Can you work these out from the model? Positions are in its coordinate system, mm. A direction names the side the tool comes from. Coordinates: 2 decimals unless noted, no trailing zeros. Write each loop counter-clockwise with the first axis right and the second up, starting at its lowest first coordinate (ties: lowest second). Pieces come first, ordered by that corner, then holes.
```python
from build123d import *

# Parameters (mm, degrees)
SKETCH1_W                      = 69.85
SKETCH1_H                      = 44.45
BOSS_EXTRUDE1_DEPTH            = 3.175
BOSS_EXTRUDE2_DEPTH            = 5.08
FILLET1_R                      = 6.35
F_6_0_204_DIAMETER_HOLE1_D     = 3.6576
F_6_0_204_DIAMETER_HOLE1_DEPTH = 38.1
F_6_0_204_DIAMETER_HOLE1_TIP   = 1.0988539


with BuildPart() as part:
    # Sketch1 → Boss-Extrude1 (new body)
    with BuildSketch(Plane(origin=(0, 0, 0), x_dir=(1, 0, 0), z_dir=(0, 1, 0))):
        Rectangle(SKETCH1_W, SKETCH1_H)
    extrude(amount=BOSS_EXTRUDE1_DEPTH)

    # Sketch2 → Boss-Extrude2 (add)
    with BuildSketch(Plane(origin=(34.925, 0, 0), x_dir=(0, 0, -1), z_dir=(1, 0, 0))):
        Polygon((-22.225, 0), (-22.225, -19.05), (-18.161, -19.05), (-18.161, -15.2219533), (-15.0040594, -12.065), (-12.681966, -12.065), (-9.525, -15.2219533), (-9.525, 0), align=None)
    extrude(amount=-BOSS_EXTRUDE2_DEPTH)

    # Fillet1
    fillet1_edges = [part.edges().sort_by_distance(p)[0] for p in [
        (-34.925, 1.5875, -22.225),
        (34.925, 1.5875, -22.225),
    ]]
    fillet(fillet1_edges, radius=FILLET1_R)

    # #6 (0.204) Diameter Hole1
    with Locations(Plane(origin=(0, 0, 0), x_dir=(-1, 0, 0), z_dir=(0, -1, 0))):
        with Locations((-29.845, 17.78), (29.845, 17.78), (31.75, -18.415), (-31.75, -5.715)):
            Hole(F_6_0_204_DIAMETER_HOLE1_D / 2, depth=F_6_0_204_DIAMETER_HOLE1_DEPTH)
            with Locations((0, 0, -(F_6_0_204_DIAMETER_HOLE1_DEPTH + F_6_0_204_DIAMETER_HOLE1_TIP / 2))):  # 118° drill point
                Cone(0, F_6_0_204_DIAMETER_HOLE1_D / 2, F_6_0_204_DIAMETER_HOLE1_TIP, mode=Mode.SUBTRACT)


solid = part.part
```
1. If we section it at A-A, the plane z = -17.78: List the corners of the cut face in (x, y) for me (3 decimals).
2. We'd pull the mould along X, two halves only. Please class faces 1 (the face through (33.02, 1.61, -20.41)), 2 (the face through (33.494, 1.61, 5.166)), 3 (the face through (-33.02, 1.61, -20.41)): released by +X, released by -X, zero draft, split by the parting line, or undercut.
3. I'm going to push flat-ended pins straight in: P1, Ø4, axis at x = 29.845, z = -17.78, coming from the -Y side; P2, Ø2.5, axis at x = 33, z = 14, coming from the -Y side; P3, Ø4, axis at y = -17, z = 12, coming from the +X side; P4, Ø10, axis at y = -10.5, z = 16, coming from the -X side (3 decimals). Where does each tip first touch, or does it pass through?
4. If we section it at B-B, the plane y = -14: List the corners of the cut face in (x, z) for me (3 decimals), plus the area to 3 significant figures.
5. If we section it at C-C, the plane x = -26: List the corners of the cut face in (y, z) for me (3 decimals), plus the area to 3 significant figures.
6. Which directions (+Z, -Z, +X, -X, +Y, -Y) give clear straight access to the entire face, cutting with the end or side of a thin tool? Please do faces 4 (the face through (29.845, -7, 16)), 5 (the face through (32, -17, 18.161)), 6 (the face through (32, -12.065, 14)), 7 (the face through (-28.86, 1.61, -19.32)).
7. If we section it at D-D, the plane y = -5.25: List the corners of the cut face in (x, z) for me (3 decimals), plus the area to 3 significant figures.
8. If I drill on L1, parallel to X at y = 1.3, z = -17.78; L2, parallel to Y at x = -21.5, z = 9 (3 decimals); L3, parallel to Z at x = 31, y = -8.5 (3 decimals), over which ranges is the centre line in solid material (lowest first)?
Answers:
1. outline: (-34.633, 0) - (-31.674, 0) - (-31.674, 3.175) - (-34.633, 3.175) - close; (-28.016, 0) - (28.016, 0) - (28.016, 3.175) - (-28.016, 3.175) - close; (31.674, 0) - (34.633, 0) - (34.633, 3.175) - (31.674, 3.175) - close
2. face 1: released by +X
2. face 2: undercut
2. face 3: released by -X
3. P1: stops at y = 0
3. P2: stops at y = -12.31
3. P3: passes through
3. P4: stops at x = 29.845
4. outline: (29.845, 9.525) - (34.925, 9.525) - (34.925, 10.747) - (29.845, 10.747) - close; (29.845, 16.939) - (34.925, 16.939) - (34.925, 22.225) - (29.845, 22.225) - close
4. area: 33.1 mm2
5. outline: (0, -22.225) - (3.175, -22.225) - (3.175, 22.225) - (0, 22.225) - close
5. area: 141 mm2
6. face 4: +Z, -Z, -X, -Y
6. face 5: -Z, +X, -X, -Y
6. face 6: +X, -X, -Y
6. face 7: +Y, -Y
7. outline: (29.845, 9.525) - (34.925, 9.525) - (34.925, 22.225) - (29.845, 22.225) - close
7. area: 64.5 mm2
8. L1: x = -34.63 to -31.67, -28.02 to 28.02, 31.67 to 34.63
8. L2: y = 0 to 3.175
8. L3: z = 9.525 to 22.225
